Drawing for the job (mm, zero at the part's lowest x, y, z). A direction names the side the tool comes from. Round coordinates to 2 decimals unless told otherwise and drop trailing zeros. Order: outer loops, then holes, each group sorted by start corner. A loop starts at its lowest first (then second) coordinate and runs counter-clockwise, first axis right, second up. Notation, with made-up numbers: M -29,24.25 L 29,24.25 A9 cw 29,31.25 Z; hole C 31,77.25 d2. An arc over 180 degrees is marked long. One line per item, written item: value. Start each with the question number.
Item 1: Pin check, flat tips, straight feed: pin 1 (4.5 mm diameter, centred on y = 8, z = 8, fed in from -X); pin 2 (4 mm diameter, centred on y = 3.5, z = 4, fed in from +X); pin 3 (1.5 mm diameter, centred on x = 3.5, z = 13, fed in from -Y); pin 4 (4 mm diameter, centred on x = 4.5, y = 8.5, fed in from +Z). Stop position of each tip, or through.
Item 2: Band-saw the part on A-A, the plane y = 5.5. Write the cut outline in (x, z).
Item 3: Probe L1, parallel to X at y = 8.75, z = 11.75 (1 decimal); L2, parallel to Z at x = 7.5, y = 6.25; L3, parallel to Y at x = 26.25, z = 3.25. List the from-to ranges inside material, lowest first.
Item 4: Band-saw the part on C-C, the plane x = 6.5. Write the cut outline in (y, z).
Item 5: Tool access for the marked faces 1, 2 and 3: list every direction of +Z, -Z, +X, -X, +Y, -Y with a clear straight run to the whole face (end or side of a thin tool).
Item 6: Band-saw the part on D-D, the plane x = 13.5. Write the cut outline in (y, z), then the cut area to 3 significant figures.
Item 7: Band-saw the part on B-B, the plane z = 3.25. Write the cut outline in (x, y).
Item 8: Two-plate mould, pull along Z, no slides. Class the marked faces 4, 5, 6 and 7: +Z half, -Z half, draft (parallel to the pull), parting line (faces both ways), or undercut.
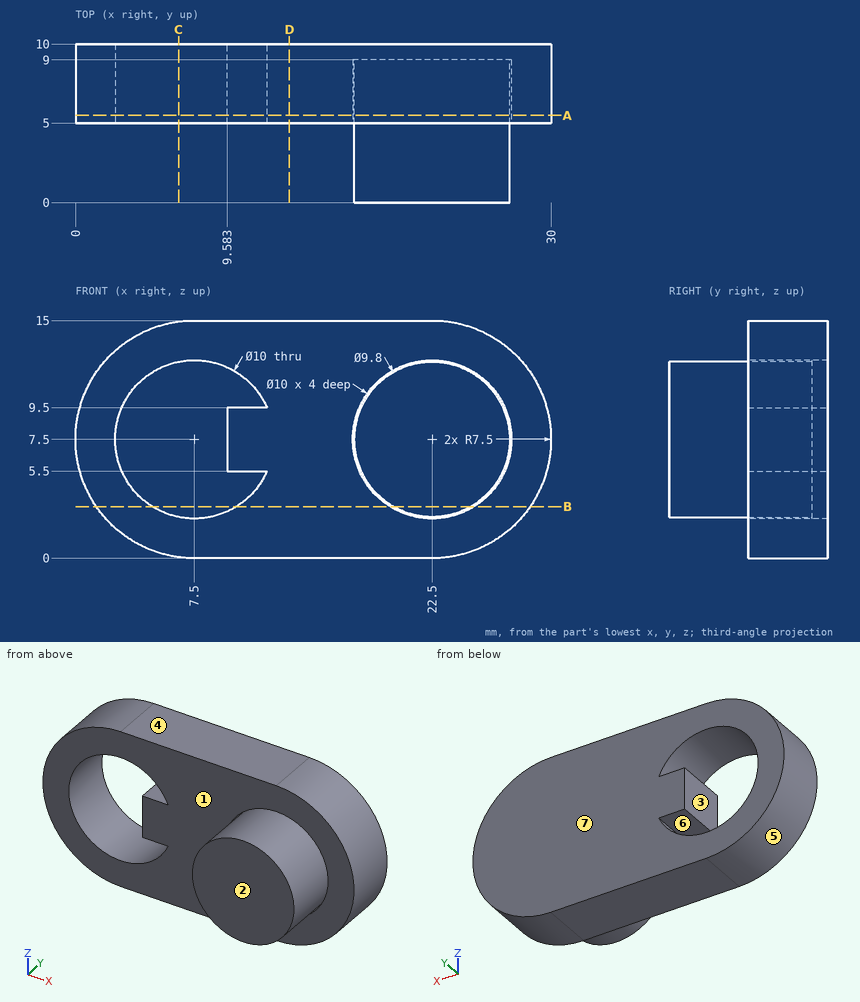
Output:
1. pin 1: stops at x = 0
1. pin 2: stops at x = 29.68
1. pin 3: stops at y = 5
1. pin 4: stops at z = 14.93
2. outline: M 7.5,0 L 22.5,0 A7.5 ccw 22.5,15 L 7.5,15 A7.5 ccw Z; C 22.5,7.5 d9.8; hole M 9.58,5.5 L 9.58,9.5 L 12.08,9.5 A5 ccw long 12.08,5.5 Z; hole C 22.5,7.5 d10
3. L1: x = 1.3 to 4.9, 10.1 to 19.9, 20.1 to 24.9, 25.1 to 28.7
3. L2: z = 0 to 2.5, 12.5 to 15
3. L3: y = 5 to 10
4. outline: M 5,0.07 L 10,0.07 L 10,2.6 L 5,2.6 Z; M 5,12.4 L 10,12.4 L 10,14.93 L 5,14.93 Z
5. face 1: -Y
5. face 2: +Z, -Z, +X, -X, -Y
5. face 3: +Y, -Y
6. outline: M 5,0 L 10,0 L 10,15 L 5,15 Z
6. area: 75.0 mm²
7. outline: M 1.32,5 L 4.87,5 L 4.87,10 L 1.32,10 Z; M 10.13,5 L 19.87,5 L 19.87,9 L 20.06,9 L 20.06,0 L 24.94,0 L 24.94,9 L 25.13,9 L 25.13,5 L 28.68,5 L 28.68,10 L 10.13,10 Z
8. face 4: +Z half
8. face 5: parting line
8. face 6: undercut
8. face 7: draft
